Verification items for the finished model (mm, model axes). Face numbers are marked on the shaded views. A direction names the side the tool comes from. Give positions to 0.01 mm unless a question says otherwise; leave off trailing zeros. Loops run counter-clockwise (first coordinate to the right, second up) from the corner with the lowest first, then second, coordinate; pieces in that order, holes last. Notation, with made-up numbers: (66.25, 65.25) - (109.25, 65.25) arc R19 ccw to (109.25, 89.25) - close; hole circle Ø8 at (32, 48.25). An arc over 180 degrees is marked (long way). Answer in a Markdown table with one row per item.
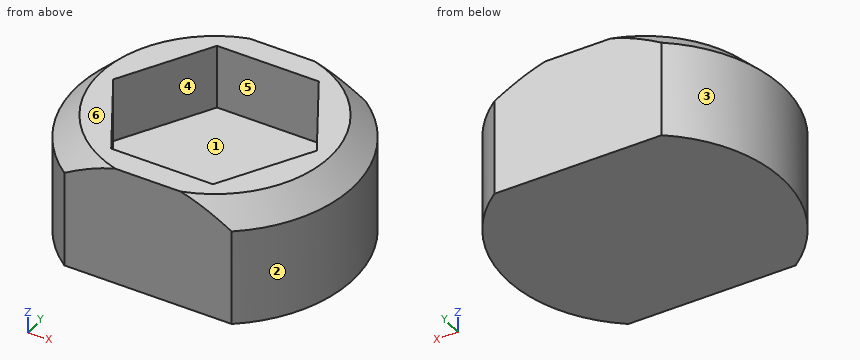
```python
from build123d import *

# Parameters (mm, degrees)
F1_DEPTH = 13
F3_DEPTH = 7
F4_SIZE  = 2.5
F5_DEPTH = 2


# Not quite as in the source:
# - a feature names something its author has since deleted; it is built from what else it names


with BuildPart() as f1:
    # F0 (on Top) → F1 (new body)
    with BuildSketch(Plane.XY):
        with BuildLine():
            ThreePointArc((9, -12), (13.416407865, -6.7082039325), (15, 0))
            ThreePointArc((15, 0), (13.416407865, 6.7082039325), (9, 12))
            Line((9, 12), (-9, 12))
            ThreePointArc((-9, 12), (-15, 0), (-9, -12))
            Line((-9, -12), (9, -12))
        make_face()
    extrude(amount=F1_DEPTH)

    # F2 (on face) → F3 (cut)
    with BuildSketch(Plane.XY.offset(13)):
        Polygon((5.4703938006, -9.475), (10.9407876011, 0), (5.4703938006, 9.475), (-5.4703938006, 9.475), (-10.9407876011, 0), (-5.4703938006, -9.475), align=None)
    extrude(amount=-F3_DEPTH, mode=Mode.SUBTRACT)

    # F4
    f4_edges = [f1.edges().sort_by_distance(p)[0] for p in [
        (15, 0, 13),
        (-15, 0, 13),
    ]]
    chamfer(f4_edges, length=F4_SIZE)

    # F0 (on Top) → F5 (join)
    with BuildSketch(Plane.XY):
        with BuildLine():
            ThreePointArc((9, -12), (13.416407865, -6.7082039325), (15, 0))
            ThreePointArc((15, 0), (13.416407865, 6.7082039325), (9, 12))
            Line((9, 12), (-9, 12))
            ThreePointArc((-9, 12), (-15, 0), (-9, -12))
            Line((-9, -12), (9, -12))
        make_face()
    extrude(amount=F5_DEPTH)


solid = f1.part
```
Q1. Tool access check on the marked faces 5 and 6. Record the directions out of +Z, -Z, +X, -X, +Y, -Y that give a thin tool (end or side, any length) a straight path to the whole face; none if there is none.
Completed:
| item | result |
|---|---|
| face 5 | +Z |
| face 6 | +Z, +X, -X, +Y, -Y |
Q2. Thickness scan on line 1 (Y direction, x = -5.25, z = 9.25) (3 decimals); line 2 (Z direction, x = -5.5, y = -9); line 3 (X direction, y = 2, z = 8.75). Record the ranges inside material, lowest first.
Completed:
| item | result |
|---|---|
| line 1 | -12 to -9.475, 9.475 to 12 |
| line 2 | 0 to 6 |
| line 3 | -14.87 to -9.79, 9.79 to 14.87 |
Q3. Go/stop test with a flat-tipped pin: P1, Ø5.5, axis at x = 0, y = 2, coming from the +Z side. Record where the tip stops, or that it passes through.
Completed:
| item | result |
|---|---|
| P1 | z = 6 |
Q4. Sectioned sample at D-D (z = 11.75). Record the cut outline in (x, y) (3 decimals), and give its area (3 significant figures).
Completed:
| item | result |
|---|---|
| outline | (-6.713, -12) - (6.713, -12) arc R13.75 ccw to (6.713, 12) - (-6.713, 12) arc R13.75 ccw to start; hole (-10.941, 0) - (-5.47, -9.475) - (5.47, -9.475) - (10.941, 0) - (5.47, 9.475) - (-5.47, 9.475) - close |
| area | 251 mm^2 |
Q5. Sectioned sample at C-C (z = 5.5). Record the cut outline in (x, y).
Completed:
| item | result |
|---|---|
| outline | (-9, -12) - (9, -12) arc R15 ccw to (9, 12) - (-9, 12) arc R15 ccw to start |
Q6. Sectioned sample at A-A (z = 7). Record the cut outline in (x, y) (3 decimals).
Completed:
| item | result |
|---|---|
| outline | (-9, -12) - (9, -12) arc R15 ccw to (9, 12) - (-9, 12) arc R15 ccw to start; hole (-10.941, 0) - (-5.47, -9.475) - (5.47, -9.475) - (10.941, 0) - (5.47, 9.475) - (-5.47, 9.475) - close |
Q7. Draft check along X on the marked faces 1, 2, 3 and 4. Enter one of: +X half, -X half, draft (parallel to the pull), parting line (faces both ways), or undercut.
Completed:
| item | result |
|---|---|
| face 1 | undercut |
| face 2 | +X half |
| face 3 | -X half |
| face 4 | undercut |
Q8. Sectioned sample at B-B (x = -1). Record the cut outline in (y, z) (3 decimals).
Completed:
| item | result |
|---|---|
| outline | (-12, 0) - (12, 0) - (12, 13) - (9.475, 13) - (9.475, 6) - (-9.475, 6) - (-9.475, 13) - (-12, 13) - close |
